from build123d import *

# Parameters (mm, degrees)
SKETCH_1_R             = 43
SKETCH_1_R_2           = 1
EXTRUDE_1_DEPTH        = 0.75
SKETCH_3_W             = 6.520751419
SKETCH_3_H             = 6.52075142
SKETCH_3_R             = 1.848339335
EXTRUDE_2_DEPTH        = 1
SKETCH_3_3_R           = 1.848339335
EXTRUDE_3_DEPTH        = 2
PATTERN_LINEAR_1_COUNT = 4
PATTERN_LINEAR_1_PITCH = 10


with BuildPart() as part:
    # Sketch 1 → Extrude 1 (new, symmetric)
    with BuildSketch(Plane(origin=(0, 0, 0), x_dir=(1, 0, 0), z_dir=(0, 1, 0))):
        with Locations(Location((0, 0, 0), (0, 0, 270))):
            Circle(SKETCH_1_R)
        with Locations(Location((-20, 20, 0), (0, 0, 270))):
            Circle(SKETCH_1_R_2, mode=Mode.SUBTRACT)
        with Locations(Location((-20, -20, 0), (0, 0, 90))):
            Circle(SKETCH_1_R_2, mode=Mode.SUBTRACT)
        with Locations(Location((20, -20, 0), (0, 0, 270))):
            Circle(SKETCH_1_R_2, mode=Mode.SUBTRACT)
        with Locations(Location((20, 20, 0), (0, 0, 90))):
            Circle(SKETCH_1_R_2, mode=Mode.SUBTRACT)
    extrude(amount=EXTRUDE_1_DEPTH, both=True)

    # Sketch 3 → Extrude 2 (add)
    with BuildSketch(Plane(origin=(0, 0.75, 0), x_dir=(1, 0, 0), z_dir=(0, 1, 0))):
        with Locations((-15.822411534, -32.507863696)):
            Rectangle(SKETCH_3_W, SKETCH_3_H)
        with Locations(Location((-15.822411533, -32.507863696, 0), (0, 0, 270))):
            Circle(SKETCH_3_R, mode=Mode.SUBTRACT)
    extrude_2 = extrude(amount=EXTRUDE_2_DEPTH)

    # Sketch 3_3 → Extrude 3 (add)
    with BuildSketch(Plane(origin=(0, 0.75, 0), x_dir=(1, 0, 0), z_dir=(0, 1, 0))):
        with Locations(Location((-15.822411533, -32.507863696, 0), (0, 0, 270))):
            Circle(SKETCH_3_3_R)
    extrude_3 = extrude(amount=EXTRUDE_3_DEPTH)

    # Pattern Linear 1: Extrude 2, Extrude 3 ×4
    with Locations(*[(i * PATTERN_LINEAR_1_PITCH, 0, 0) for i in range(1, PATTERN_LINEAR_1_COUNT)]):
        add(extrude_2)
        add(extrude_3)


solid = part.part
Read the model definition and answer for the solid it produces. Units are mm, in the model's axes. A direction names the side the tool comes from. Give positions to 0.01 mm unless a question says otherwise; leave off trailing zeros. Loops run counter-clockwise (first coordinate to the right, second up) from the corner with the lowest first, then second, coordinate; pieces in that order, holes last. Notation, with made-up numbers: (-23, -15) - (10, -15) arc R11 ccw to (10, -3) - close; hole circle Ø11 at (28.5, 50). An arc over 180 degrees is marked (long way). Answer as CSV lines item,"result". Start each with the question number.
1) Straight lines are drawn through the part: L1, parallel to X at y = -0.2, z = -20; L2, parallel to Y at x = 5, z = 19.5; L3, parallel to X at y = 0.4, z = 0. For each, find the intervals that lie inside material, in ascending order. Write a range as from..to.
2) Find section C-C (z = 0). Write down the section's boundary in (x, y), then the cut area to 3 significant figures.
3) Determine the mould class of faces 1 (the face through (3.47, 2.243, 34.215)), 2 (the face through (-16, 2.75, 32)), 3 (the face through (29.061, 0.01, -31.693)) for opening direction X: released by +X, released by -X, zero draft, split by the parting line, or undercut.
4) Each of these flat-tipped pins is pushed along its axis until it touches: pin 1 Ø0.5 at (y, z) = (1.5, 31.5) entering from +X; pin 2 Ø6 at (x, z) = (11, -28) entering from +Y; pin 3 Ø0.8 at (x, y) = (-16, 1) entering from -Z; pin 4 Ø1.2 at (x, z) = (20, -20) entering from +Y (3 decimals). Where does it stop, or does it pass through?
5) Find section D-D (x = -30). Write down the section's boundary in (y, z).
6) Find section A-A (x = 20). Write down the section's boundary in (y, z).
7) Which of the six approach directions +Z, -Z, +X, -X, +Y, -Y give full straight-line access (tool end or side, diameter ignored) to faces 4 (the face through (19, 0, 20)), 5 (the face through (-6.53, 2.243, 34.215))?
8) Find section B-B (z = -20). Write down the section's boundary in (x, y).
Findings below:
1,L1,"-38.07..-21, -19..19, 21..38.07"
1,L2,"-0.75..0.75"
1,L3,"-43..43"
2,outline,"(-43, -0.75) - (43, -0.75) - (43, 0.75) - (-43, 0.75) - close"
2,area,"129 mm^2"
3,face 1,"undercut"
3,face 2,"zero draft"
3,face 3,"split by the parting line"
4,pin 1,"x = 17.44"
4,pin 2,"y = 0.75"
4,pin 3,"z = -40.04"
4,pin 4,"through"
5,outline,"(-0.75, -30.81) - (0.75, -30.81) - (0.75, 30.81) - (-0.75, 30.81) - close"
6,outline,"(-0.75, -38.07) - (0.75, -38.07) - (0.75, -21) - (-0.75, -21) - close; (-0.75, -19) - (0.75, -19) - (0.75, 19) - (-0.75, 19) - close; (-0.75, 21) - (0.75, 21) - (0.75, 38.07) - (-0.75, 38.07) - close"
7,face 4,"+Y, -Y"
7,face 5,"+Y"
8,outline,"(-38.07, -0.75) - (-21, -0.75) - (-21, 0.75) - (-38.07, 0.75) - close; (-19, -0.75) - (19, -0.75) - (19, 0.75) - (-19, 0.75) - close; (21, -0.75) - (38.07, -0.75) - (38.07, 0.75) - (21, 0.75) - close"
